Check sheet for the modelled part. Datum: model origin and axes. Units: mm. Face numbers are marked on the shaded views. A direction names the side the tool comes from. Give positions to 0.01 mm unless a question says otherwise; leave off trailing zeros. Order: outer loops, then holes, each group sorted by start corner. A loop starts at its lowest first (then second) coordinate and runs counter-clockwise, first axis right, second up. Notation, with made-up numbers: (75.5, 77) - (105.5, 77) arc R14 cw to (105.5, 93) - close; hole circle Ø11 at (40, -7). An arc over 180 degrees is marked (long way). Answer in a Markdown table with one row per item.
from build123d import *

# Parameters (mm, degrees)
F0_W        = 20
F0_H        = 2.5
F1_DEPTH    = 9.2
F2_DEPTH    = 10
F3_R        = 2
F4_DEPTH    = 25
F5_W        = 1
F5_H        = 6.7
F6_DEPTH    = 0.8
F7_T1_DEPTH = 10
F7_T6_DEPTH = 20.3706815716
F8_ANGLE    = 180


# Not quite as in the source:
# - a fillet or chamfer that OpenCascade refuses, or shapes differently, is made with other operations: its cross-section is extruded or revolved along the edge and cut away or added


with BuildPart() as f1:
    # F0 (on Top) → F1 (new body)
    with BuildSketch(Plane.XY):
        Polygon((-9.1, -3.35), (-10.1, -3.35), (-10.1, 3.35), (10.1, 3.35), (10.1, -3.35), (9.1, -3.35), (9.1, -4.95), (11.7, -4.95), (11.7, 3.35), (11.7, 7.35), (10.8, 7.35), (-11.7, 7.35), (-11.7, -4.95), (-9.1, -4.95), align=None)
        Polygon((13.3, 7.35), (11.7, 7.35), (11.7, 3.35), (13.3, 3.35), (13.3, 5.85), align=None)
        Polygon((13.3, 9.85), (10.8, 7.35), (11.7, 7.35), (13.3, 7.35), align=None)
        with Locations((23.3, 8.6)):
            Rectangle(F0_W, F0_H)
        Polygon((33.3, 7.35), (13.3, 7.35), (13.3, 5.85), (15.8, 5.85), (33.3, 5.85), align=None)
        Polygon((13.3, 5.85), (13.3, 3.35), (15.8, 5.85), align=None)
    extrude(amount=F1_DEPTH)

    # F0 (on Top) → F2 (join, symmetric)
    with BuildSketch(Plane.XY):
        Polygon((33.3, 7.35), (13.3, 7.35), (13.3, 5.85), (15.8, 5.85), (33.3, 5.85), align=None)
        with Locations((23.3, 8.6)):
            Rectangle(F0_W, F0_H)
    extrude(amount=F2_DEPTH, both=True)

    # F3 (on face) → F4 (cut)
    with BuildSketch(Plane.XZ.offset(-5.85)):
        with Locations((23.3, 5)):
            Circle(F3_R)
        with Locations((23.3, -5)):
            Circle(F3_R)
    extrude(amount=-F4_DEPTH, mode=Mode.SUBTRACT)

    # F5 (on face) → F6 (join, through all)
    with BuildSketch(Plane.XY.offset(9.2)):
        Polygon((-9.1, -4.95), (-9.1, -3.35), (-10.1, -3.35), (-10.1, 3.35), (-9.1, 3.35), (9.1, 3.35), (10.1, 3.35), (10.1, -3.35), (9.1, -3.35), (9.1, -4.95), (11.7, -4.95), (11.7, 3.35), (13.3, 3.35), (15.8, 5.85), (13.3, 5.85), (13.3, 9.85), (10.8, 7.35), (-11.7, 7.35), (-11.7, -4.95), align=None)
        with Locations((-9.6, 0)):
            Rectangle(F5_W, F5_H)
        with Locations((9.6, 0)):
            Rectangle(F5_W, F5_H)
    extrude(amount=F6_DEPTH)

    # F7: chamfer of 2 on 2 edges, made by hand

    # F7_s2 → F7_t1 (join)
    with BuildSketch(Plane.XY):
        Polygon((12.2142135624, 8.7642135624), (8.8, 7.35), (10.8, 7.35), align=None)
    extrude(amount=F7_T1_DEPTH)


with BuildPart() as f7_tool4:
    # F7_s5 → F7_t6 (new body)
    with BuildSketch(Plane.XY.offset(15.1853407858)):
        Polygon((11.3, 3.35), (14.7142135624, 4.7642135624), (13.3, 3.35), align=None)
    extrude(amount=-F7_T6_DEPTH)

    split(bisect_by=Plane.YZ.offset(11.7), keep=Keep.TOP)


with BuildPart() as f1_1:
    add(f1.part)

    # F7_t3: cut F7_tool4
    add(f7_tool4.part, mode=Mode.SUBTRACT)


with BuildPart() as f1_2:
    # F8: moved
    add(f1_1.part.rotate(Axis((24.55, 5.85, 10), (1, 0, 0)), F8_ANGLE))


solid = f1_2.part
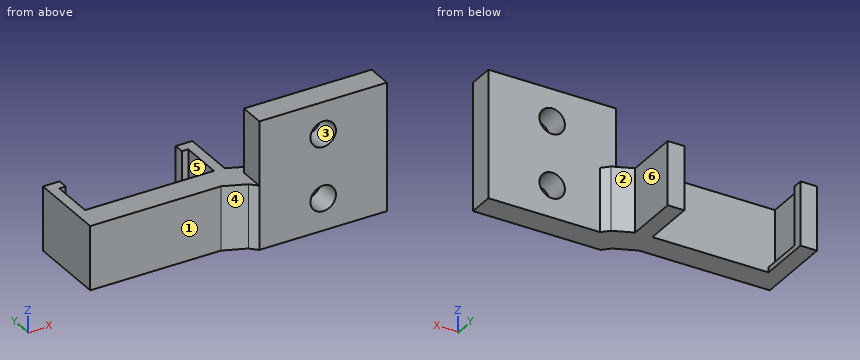
(1) Access from +Z, -Z, +X, -X, +Y, -Y to the whole of each face (thin tool, end or side, straight path). Record for the marked faces 4, 5 and 6.
Geometry says:
| item | result |
|---|---|
| face 4 | +Z, -Z, -X, -Y |
| face 5 | +Z |
| face 6 | +Z, -Z, +X, +Y |
(2) Mould release check, pull along X, two halves, no side actions. Record for the marked faces 1, 2 and 3: pulls with the +X half, pulls with the -X half, needs draft (parallel to the pull), parting line crosses it, or undercut.
Geometry says:
| item | result |
|---|---|
| face 1 | needs draft |
| face 2 | pulls with the +X half |
| face 3 | undercut |
(3) Cross-section at C-C, the plane x = 23.3. Record the cut outline in (y, z), then the cut area to 3 significant figures.
Geometry says:
| item | result |
|---|---|
| outline | (1.85, 10) - (5.85, 10) - (5.85, 13) - (1.85, 13) - close; (1.85, 17) - (5.85, 17) - (5.85, 23) - (1.85, 23) - close; (1.85, 27) - (5.85, 27) - (5.85, 30) - (1.85, 30) - close |
| area | 48.0 mm² |
(4) Cross-section at B-B, the plane y = 13.25. Record the cut outline in (x, z).
Geometry says:
| item | result |
|---|---|
| outline | (-11.7, 10) - (-9.1, 10) - (-9.1, 10.8) - (-10.1, 10.8) - (-10.1, 20) - (-11.7, 20) - close; (9.1, 10) - (11.7, 10) - (11.7, 20) - (10.1, 20) - (10.1, 10.8) - (9.1, 10.8) - close |
(5) Cross-section at A-A, the plane z = 15. Record the cut outline in (x, y).
Geometry says:
| item | result |
|---|---|
| outline | (-11.7, 4.35) - (8.8, 4.35) - (12.21, 2.94) - (13.3, 1.85) - (21.3, 1.85) - (21.3, 5.85) - (15.8, 5.85) - (14.71, 6.94) - (11.7, 8.18) - (11.7, 16.65) - (9.1, 16.65) - (9.1, 15.05) - (10.1, 15.05) - (10.1, 8.35) - (-10.1, 8.35) - (-10.1, 15.05) - (-9.1, 15.05) - (-9.1, 16.65) - (-11.7, 16.65) - close; (25.3, 1.85) - (33.3, 1.85) - (33.3, 5.85) - (25.3, 5.85) - close |
(6) Cross-section at D-D, the plane z = 18.5. Record the cut outline in (x, y).
Geometry says:
| item | result |
|---|---|
| outline | (-11.7, 4.35) - (8.8, 4.35) - (12.21, 2.94) - (13.3, 1.85) - (33.3, 1.85) - (33.3, 5.85) - (15.8, 5.85) - (14.71, 6.94) - (11.7, 8.18) - (11.7, 16.65) - (9.1, 16.65) - (9.1, 15.05) - (10.1, 15.05) - (10.1, 8.35) - (-10.1, 8.35) - (-10.1, 15.05) - (-9.1, 15.05) - (-9.1, 16.65) - (-11.7, 16.65) - close |
(7) Thickness scan on L1, parallel to Z at x = 23.3, y = 2.95; L2, parallel to X at y = 3.8, z = 25; L3, parallel to X at y = 14, z = 13.75. Record the ranges inside material, lowest first.
Geometry says:
| item | result |
|---|---|
| L1 | 10 to 13, 17 to 23, 27 to 30 |
| L2 | 13.3 to 21.3, 25.3 to 33.3 |
| L3 | -11.7 to -10.1, 10.1 to 11.7 |
(8) Gauge pin test, flat ends, axial feed: P1, Ø4.5, axis at x = 23.3, z = 25, coming from the +Y side; P2, Ø7, axis at y = 12.5, z = 15.5, coming from the +X side; P3, Ø7.5, axis at x = 5.5, y = 13, coming from the +Z side. Record the tip position at first contact, or that the pin passes through.
Geometry says:
| item | result |
|---|---|
| P1 | y = 5.85 |
| P2 | x = 11.7 |
| P3 | z = 10.8 |
